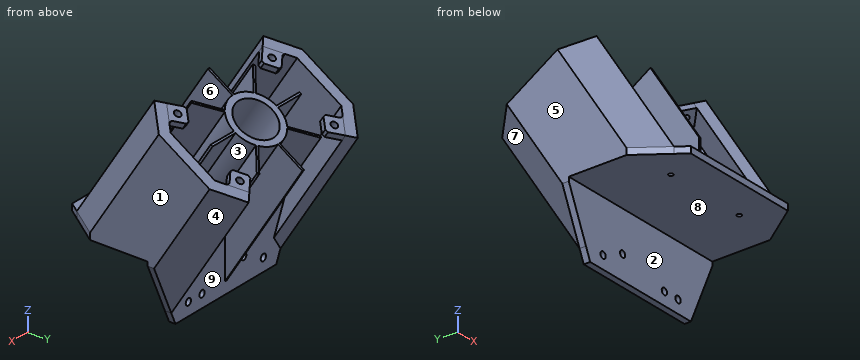
```python
from build123d import *

# Parameters (mm, degrees)
BOSS_EXTRUDE1_DEPTH = 3
SKETCH3_W           = 84
SKETCH3_H           = 3
BOSS_EXTRUDE2_DEPTH = 30
BOSS_EXTRUDE3_DEPTH = 68
SKETCH8_R           = 9.5
BOSS_EXTRUDE4_DEPTH = 68
SKETCH9_W           = 30
SKETCH9_H           = 46
CUT_EXTRUDE3_DEPTH  = 85
CUT_EXTRUDE4_DEPTH  = 68
CUT_EXTRUDE5_DEPTH  = 68
BOSS_EXTRUDE5_DEPTH = 8
CHAMFER1_SIZE       = 1
BOSS_EXTRUDE6_DEPTH = 8
CHAMFER2_SIZE       = 1
BOSS_EXTRUDE7_DEPTH = 8
CHAMFER3_SIZE       = 1
BOSS_EXTRUDE8_DEPTH = 8
CHAMFER4_SIZE       = 1
CUT_EXTRUDE6_REACH  = 100.635
SKETCH17_R          = 1.55
CUT_EXTRUDE7_REACH  = 51
SKETCH18_R          = 1.55
SKETCH18_R_2        = 1.5
SKETCH21_W          = 45
SKETCH21_H          = 22
CUT_EXTRUDE8_DEPTH  = 58.667270539
SKETCH22_R          = 1.05
CUT_EXTRUDE9_DEPTH  = 3


with BuildPart() as part:
    # Sketch2 → Boss-Extrude1 (new body)
    with BuildSketch(Plane.XY):
        Polygon((-110, 46), (-110, 49), (-26, 49), (-26, 46), (-26, 0), (-110, 0), align=None)
    extrude(amount=BOSS_EXTRUDE1_DEPTH)

    # Sketch3 → Boss-Extrude2 (add)
    with BuildSketch(Plane(origin=(0, 0, 0), x_dir=(-1, 0, 0), z_dir=(0, 0, -1))):
        with Locations((68, 47.5)):
            Rectangle(SKETCH3_W, SKETCH3_H)
    extrude(amount=BOSS_EXTRUDE2_DEPTH)

    # Sketch7 → Boss-Extrude3 (add)
    with BuildSketch(Plane(origin=(0, 2.752263202, 4.404541836), x_dir=(1, 0, 0), z_dir=(0, 0.529919264, 0.848048096))):
        Polygon((-110, 14.650482688), (-99.930804426, 2.650482688), (-96.10058221, 5.864420737), (-105, 16.470333859), (-105, 40.714481265), (-96.10058221, 51.320394388), (-99.930804426, 54.534332436), (-110, 42.534332436), align=None)
        Polygon((-39.89941779, 5.864420737), (-36.069195574, 2.650482688), (-26, 14.650482688), (-26, 39.964598919), (-26, 42.534332436), (-36.069195574, 54.534332436), (-39.89941779, 51.320394388), (-31, 40.714481265), (-31, 16.470333859), align=None)
    extrude(amount=BOSS_EXTRUDE3_DEPTH)

    # Sketch8 → Boss-Extrude4 (add)
    with BuildSketch(Plane(origin=(0, 2.752263202, 4.404541836), x_dir=(1, 0, 0), z_dir=(0, 0.529919264, 0.848048096))):
        with BuildLine():
            Line((-67.5, 54.534332436), (-68.5, 54.534332436))
            Line((-68.5, 54.534332436), (-68.5, 41.082403559))
            ThreePointArc((-68.5, 41.082403559), (-72.822037178, 40.124881601), (-76.539295111, 37.720958324))
            Line((-76.539295111, 37.720958324), (-85.990157605, 47.289671948))
            Line((-85.990157605, 47.289671948), (-86.697264386, 46.582565167))
            Line((-86.697264386, 46.582565167), (-77.185314257, 37.070615038))
            ThreePointArc((-77.185314257, 37.070615038), (-79.564385784, 33.337402971), (-80.493053625, 29.009074229))
            Line((-80.493053625, 29.009074229), (-93.941924874, 29.092407562))
            Line((-93.941924874, 29.092407562), (-93.941924874, 28.092407562))
            Line((-93.941924874, 28.092407562), (-80.489995997, 28.092407562))
            ThreePointArc((-80.489995997, 28.092407562), (-79.532474039, 23.770370384), (-77.128550762, 20.053112451))
            Line((-77.128550762, 20.053112451), (-86.697264386, 10.602249957))
            Line((-86.697264386, 10.602249957), (-85.990157605, 9.895143176))
            Line((-85.990157605, 9.895143176), (-76.478207476, 19.407093305))
            ThreePointArc((-76.478207476, 19.407093305), (-72.744995409, 17.028021778), (-68.416666667, 16.099353937))
            Line((-68.416666667, 16.099353937), (-68.5, 2.650482688))
            Line((-68.5, 2.650482688), (-67.5, 2.650482688))
            Line((-67.5, 2.650482688), (-67.5, 16.102411565))
            ThreePointArc((-67.5, 16.102411565), (-63.177962822, 17.059933523), (-59.460704889, 19.4638568))
            Line((-59.460704889, 19.4638568), (-50.009842395, 9.895143176))
            Line((-50.009842395, 9.895143176), (-49.302735614, 10.602249957))
            Line((-49.302735614, 10.602249957), (-58.814685743, 20.114200086))
            ThreePointArc((-58.814685743, 20.114200086), (-56.435614216, 23.847412153), (-55.506946375, 28.175740895))
            Line((-55.506946375, 28.175740895), (-42.058075126, 28.092407562))
            Line((-42.058075126, 28.092407562), (-42.058075126, 29.092407562))
            Line((-42.058075126, 29.092407562), (-55.510004003, 29.092407562))
            ThreePointArc((-55.510004003, 29.092407562), (-56.467525961, 33.41444474), (-58.871449238, 37.131702673))
            Line((-58.871449238, 37.131702673), (-49.302735614, 46.582565167))
            Line((-49.302735614, 46.582565167), (-50.009842395, 47.289671948))
            Line((-50.009842395, 47.289671948), (-59.521792524, 37.777721819))
            ThreePointArc((-59.521792524, 37.777721819), (-63.255004591, 40.156793346), (-67.583333333, 41.085461188))
            Line((-67.583333333, 41.085461188), (-67.5, 54.534332436))
        make_face()
        with Locations((-68, 28.592407562)):
            Circle(SKETCH8_R, mode=Mode.SUBTRACT)
    extrude(amount=BOSS_EXTRUDE4_DEPTH)

    # Sketch9 → Cut-Extrude3 (cut, through all)
    with BuildSketch(Plane.ZY.offset(110)):
        with Locations((-15, 23)):
            Rectangle(SKETCH9_W, SKETCH9_H)
    extrude(amount=-CUT_EXTRUDE3_DEPTH, mode=Mode.SUBTRACT)

    # Sketch11 → Cut-Extrude4 (cut)
    with BuildSketch(Plane(origin=(0, 49, 0), x_dir=(1, 0, 0), z_dir=(0, 1, 0))):
        Polygon((-26, 1.849292506), (-36.069195574, 24.494251484), (-38.517354506, 30), (-26, 30), align=None)
        Polygon((-110, 1.849292506), (-99.930804426, 24.494251484), (-97.482645494, 30), (-110, 30), align=None)
    extrude(amount=-CUT_EXTRUDE4_DEPTH, mode=Mode.SUBTRACT)

    # Sketch12 → Cut-Extrude5 (cut)
    with BuildSketch(Plane.XY.offset(3)):
        Polygon((-110, 19.15014084), (-99.930804426, 5), (-96.372820202, 0), (-110, 0), align=None)
        Polygon((-26, 19.15014084), (-36.069195574, 5), (-39.627179798, 0), (-26, 0), align=None)
    extrude(amount=-CUT_EXTRUDE5_DEPTH, mode=Mode.SUBTRACT)

    # Sketch13 → Boss-Extrude5 (add)
    with BuildSketch(Plane(origin=(-81.664497732, 58.112198911, -36.312532071), x_dir=(0.277530914, -0.197490123, -0.940199045), z_dir=(0.766044443, -0.545114809, 0.340625537))):
        Polygon((-75.716604077, 11.344887623), (-73.010640587, 10.049603257), (-76.464732228, 2.833700616), (-79.170695719, 4.128984981), align=None)
    extrude(amount=BOSS_EXTRUDE5_DEPTH)

    # Chamfer1
    chamfer1_edges = [part.edges().sort_by_distance(p)[0] for p in [
        (-101.242883088, 76.316916776, 36.851608258),
        (-95.114527543, 71.955998307, 39.576612555),
        (-89.972226665, 77.153138559, 36.329078894),
    ]]
    chamfer(chamfer1_edges, length=CHAMFER1_SIZE)

    # Sketch14 → Boss-Extrude6 (add)
    with BuildSketch(Plane(origin=(-53.506473088, -38.075037421, 23.791923957), x_dir=(-0.277530914, -0.197490123, -0.940199045), z_dir=(0.766044443, 0.545114809, -0.340625537))):
        Polygon((-37.409332735, 91.372162271), (-34.703369245, 90.076877905), (-31.249277603, 97.292780547), (-33.955241094, 98.588064912), align=None)
    extrude(amount=BOSS_EXTRUDE6_DEPTH)

    # Chamfer2
    chamfer2_edges = [part.edges().sort_by_distance(p)[0] for p in [
        (-101.242883088, 48.162345367, 54.444537047),
        (-89.972226665, 47.326123584, 54.967066411),
        (-95.114527543, 52.523263836, 51.71953275),
    ]]
    chamfer(chamfer2_edges, length=CHAMFER2_SIZE)

    # Sketch15 → Boss-Extrude7 (add)
    with BuildSketch(Plane(origin=(1.856421651, 1.321023789, -0.825467279), x_dir=(0.277530914, 0.197490123, 0.940199045), z_dir=(-0.766044443, -0.545114809, 0.340625537))):
        Polygon((37.972399808, 90.195865404), (35.266436317, 88.900581038), (38.720527959, 81.684678396), (41.426491449, 82.979962762), align=None)
    extrude(amount=BOSS_EXTRUDE7_DEPTH)

    # Chamfer3
    chamfer3_edges = [part.edges().sort_by_distance(p)[0] for p in [
        (-34.757116912, 76.316916776, 36.851608258),
        (-46.027773335, 77.153138559, 36.329078894),
        (-40.885472457, 71.955998307, 39.576612555),
    ]]
    chamfer(chamfer3_edges, length=CHAMFER3_SIZE)

    # Sketch16 → Boss-Extrude8 (add)
    with BuildSketch(Plane(origin=(-26.301602994, 18.716137701, -11.695140835), x_dir=(-0.277530914, 0.197490123, 0.940199045), z_dir=(-0.766044443, 0.545114809, -0.340625537))):
        Polygon((75.153537005, 12.52118449), (72.447573514, 11.225900124), (68.993481872, 18.441802766), (71.699445363, 19.737087131), align=None)
    extrude(amount=BOSS_EXTRUDE8_DEPTH)

    # Chamfer4
    chamfer4_edges = [part.edges().sort_by_distance(p)[0] for p in [
        (-34.757116912, 48.162345367, 54.444537047),
        (-40.885472457, 52.523263836, 51.71953275),
        (-46.027773335, 47.326123584, 54.967066411),
    ]]
    chamfer(chamfer4_edges, length=CHAMFER4_SIZE)

    # Sketch17 → Cut-Extrude6 (cut, up to next)
    with BuildSketch(Plane(origin=(0, 38.78677317, 62.071812375), x_dir=(1, 0, 0), z_dir=(0, 0.529919264, 0.848048096)), mode=Mode.PRIVATE) as cut_extrude6_sk1:
        with Locations((-95.607554877, 45.685066176)):
            Circle(SKETCH17_R)
    cut_extrude6_tool1 = extrude(cut_extrude6_sk1.sketch, amount=-CUT_EXTRUDE6_REACH, mode=Mode.PRIVATE) & part.part
    add(cut_extrude6_tool1.solids().sort_by_distance((-95.607555, 77.529907, 37.862416))[0], mode=Mode.SUBTRACT)
    # Sketch17 → Cut-Extrude6 (cut, up to next)
    with BuildSketch(Plane(origin=(0, 38.78677317, 62.071812375), x_dir=(1, 0, 0), z_dir=(0, 0.529919264, 0.848048096)), mode=Mode.PRIVATE) as cut_extrude6_sk2:
        with Locations((-95.607554877, 11.499748948)):
            Circle(SKETCH17_R)
    cut_extrude6_tool2 = extrude(cut_extrude6_sk2.sketch, amount=-CUT_EXTRUDE6_REACH, mode=Mode.PRIVATE) & part.part
    add(cut_extrude6_tool2.solids().sort_by_distance((-95.607555, 48.539113, 55.977874))[0], mode=Mode.SUBTRACT)
    # Sketch17 → Cut-Extrude6 (cut, up to next)
    with BuildSketch(Plane(origin=(0, 38.78677317, 62.071812375), x_dir=(1, 0, 0), z_dir=(0, 0.529919264, 0.848048096)), mode=Mode.PRIVATE) as cut_extrude6_sk3:
        with Locations((-40.392445123, 45.685066176)):
            Circle(SKETCH17_R)
    cut_extrude6_tool3 = extrude(cut_extrude6_sk3.sketch, amount=-CUT_EXTRUDE6_REACH, mode=Mode.PRIVATE) & part.part
    add(cut_extrude6_tool3.solids().sort_by_distance((-40.392445, 77.529907, 37.862416))[0], mode=Mode.SUBTRACT)
    # Sketch17 → Cut-Extrude6 (cut, up to next)
    with BuildSketch(Plane(origin=(0, 38.78677317, 62.071812375), x_dir=(1, 0, 0), z_dir=(0, 0.529919264, 0.848048096)), mode=Mode.PRIVATE) as cut_extrude6_sk4:
        with Locations((-40.392445123, 11.499748948)):
            Circle(SKETCH17_R)
    cut_extrude6_tool4 = extrude(cut_extrude6_sk4.sketch, amount=-CUT_EXTRUDE6_REACH, mode=Mode.PRIVATE) & part.part
    add(cut_extrude6_tool4.solids().sort_by_distance((-40.392445, 48.539113, 55.977874))[0], mode=Mode.SUBTRACT)

    # Sketch18 → Cut-Extrude7 (cut, up to next)
    with BuildSketch(Plane(origin=(0, 49, 0), x_dir=(1, 0, 0), z_dir=(0, 1, 0)), mode=Mode.PRIVATE) as cut_extrude7_sk1:
        with Locations((-89.930804426, 24)):
            Circle(SKETCH18_R)
    cut_extrude7_tool1 = extrude(cut_extrude7_sk1.sketch, amount=-CUT_EXTRUDE7_REACH, mode=Mode.PRIVATE) & part.part
    add(cut_extrude7_tool1.solids().sort_by_distance((-89.930804, 49, -24))[0], mode=Mode.SUBTRACT)
    # Sketch18 → Cut-Extrude7 (cut, up to next)
    with BuildSketch(Plane(origin=(0, 49, 0), x_dir=(1, 0, 0), z_dir=(0, 1, 0)), mode=Mode.PRIVATE) as cut_extrude7_sk2:
        with Locations((-54.069195574, 24)):
            Circle(SKETCH18_R)
    cut_extrude7_tool2 = extrude(cut_extrude7_sk2.sketch, amount=-CUT_EXTRUDE7_REACH, mode=Mode.PRIVATE) & part.part
    add(cut_extrude7_tool2.solids().sort_by_distance((-54.069196, 49, -24))[0], mode=Mode.SUBTRACT)
    # Sketch18 → Cut-Extrude7 (cut, up to next)
    with BuildSketch(Plane(origin=(0, 49, 0), x_dir=(1, 0, 0), z_dir=(0, 1, 0)), mode=Mode.PRIVATE) as cut_extrude7_sk3:
        with Locations((-46.069195574, 24)):
            Circle(SKETCH18_R)
    cut_extrude7_tool3 = extrude(cut_extrude7_sk3.sketch, amount=-CUT_EXTRUDE7_REACH, mode=Mode.PRIVATE) & part.part
    add(cut_extrude7_tool3.solids().sort_by_distance((-46.069196, 49, -24))[0], mode=Mode.SUBTRACT)
    # Sketch18 → Cut-Extrude7 (cut, up to next)
    with BuildSketch(Plane(origin=(0, 49, 0), x_dir=(1, 0, 0), z_dir=(0, 1, 0)), mode=Mode.PRIVATE) as cut_extrude7_sk4:
        with Locations((-78.5, 18.8)):
            Circle(SKETCH18_R_2)
    cut_extrude7_tool4 = extrude(cut_extrude7_sk4.sketch, amount=-CUT_EXTRUDE7_REACH, mode=Mode.PRIVATE) & part.part
    add(cut_extrude7_tool4.solids().sort_by_distance((-78.5, 49, -18.8))[0], mode=Mode.SUBTRACT)

    # Sketch21 → Cut-Extrude8 (cut, through all)
    with BuildSketch(Plane.XY.offset(3)):
        with Locations((-68, 7.45)):
            Rectangle(SKETCH21_W, SKETCH21_H)
    extrude(amount=CUT_EXTRUDE8_DEPTH, mode=Mode.SUBTRACT)

    # Sketch22 → Cut-Extrude9 (cut)
    with BuildSketch(Plane.XY.offset(3)):
        with Locations((-48, -1.05)):
            Circle(SKETCH22_R)
        with Locations((-88, -1.05)):
            Circle(SKETCH22_R)
        with Locations((-88, 15.95)):
            Circle(SKETCH22_R)
        with Locations((-48, 15.95)):
            Circle(SKETCH22_R)
    extrude(amount=-CUT_EXTRUDE9_DEPTH, mode=Mode.SUBTRACT)


solid = part.part
```
The listing builds one solid part. Answer for the finished solid, in the listing's coordinates (mm). Face numbers are marked on the shaded views. A direction names the side the tool comes from. Give positions to 0.01 mm unless a question says otherwise; leave off trailing zeros. Order: outer loops, then holes, each group sorted by start corner. A loop starts at its lowest first (then second) coordinate and runs counter-clockwise, first axis right, second up. Notation, with made-up numbers: M 89,30 L 142,30 A18 ccw 142,54 Z; hole C 34.5,70.5 d4. An arc over 180 degrees is marked long. Put each result on its own line as item: value. Start each with the question number.
Item 1: For a pull along Y with two mould halves and no side action, classify the marked faces 1, 2, 3 and 4 as +Y half, -Y half, draft (parallel to the pull), parting line (faces both ways), or undercut.
Item 2: The part is cut by section C-C, the plane x = -66. Determine the outline of the cut face in (y, z), and give its area (3 significant figures).
Item 3: The part is cut by section A-A, the plane z = 15. State how many separate pieces and enclosed holes the cut face has, and give its area (3 significant figures).
Item 4: Which of the six approach directions +Z, -Z, +X, -X, +Y, -Y give full straight-line access (tool end or side, diameter ignored) to the marked faces 5, 6, 7, 8 and 9?
Item 5: The part is cut by section D-D, the plane z = -6. Determine the outline of the cut face in (x, y).
Item 6: Flat-ended cylindrical pins translate along their axes: P1, Ø1.1, axis at x = -68, z = 18, coming from the -Y side; P2, Ø8, axis at y = 49, z = -14, coming from the +X side; P3, Ø10, axis at x = -72.5, z = 26.5, coming from the +Y side; P4, Ø1.9, axis at x = -54.07, z = -24, coming from the -Y side. Find the tip coordinate at first contact, or state that the pin passes through.
Item 7: Find the intervals of material crossed by line 1 along X through (y, z) = (57.5, -6.5); line 2 along X through (y, z) = (48.45, -24); line 3 along Y through (x, z) = (-88, 1.55), in increasing order.
Answer key:
1. face 1: draft
1. face 2: -Y half
1. face 3: undercut
1. face 4: +Y half
2. outline: M 0,0 L 46,0 L 46,-30 L 49,-30 L 49,1.18 L 73.5,40.38 L 70.91,42 L 46.54,3 L 24.64,3 L 55.16,51.84 L 52.57,53.46 L 21.04,3 L 0,3 Z
2. area: 554 mm²
3. separate pieces: 3
3. enclosed holes: 1
3. area: 1,020 mm²
4. face 5: +Z, -Z, -X, +Y, -Y
4. face 6: +Z, -Y
4. face 7: -Z, -X, +Y
4. face 8: -Z, +X, -X, -Y
4. face 9: none
5. outline: M -108.15,46 L -27.85,46 L -27.85,49 L -36.07,60.56 L -39.9,56.77 L -34.37,49 L -51.17,49 L -49.3,51.18 L -50.01,52.01 L -52.57,49 L -67.56,49 L -67.5,60.56 L -68.5,60.56 L -68.5,49 L -83.47,49 L -85.99,52.01 L -86.7,51.18 L -84.85,49 L -101.63,49 L -96.1,56.77 L -99.93,60.56 L -108.15,49 Z
6. P1: stops at y = 18.45
6. P2: stops at x = -29.62
6. P3: stops at y = 82.74
6. P4: passes through
7. line 1: x = -101.88 to -97.16, -68.5 to -67.51, -38.84 to -34.12
7. line 2: x = -100.15 to -91.48, -88.38 to -55.62, -52.52 to -47.62, -44.52 to -35.85
7. line 3: y = 0 to 14.9, 17 to 49
